Could you check a few things on this model? Use its own coordinates, in mm. Coordinates: 2 decimals unless noted, no trailing zeros. Loops run counter-clockwise (first coordinate to the right, second up) from the corner with the lowest first, then second, coordinate; pieces in that order, holes last. Notation, with made-up numbers: (39.25, 28.5) - (65.25, 28.5) arc R25 cw to (65.25, 66.5) - close; hole circle Ø1 at (70, -34.75). An arc over 180 degrees is marked (long way). One line per question, with ' | ' between items. Start each with the question number.
1. Please list where these lines run through material, in increasing order: L1, parallel to X at y = 8.5, z = 1.3; L2, parallel to X at y = -9, z = 1; L3, parallel to X at y = -1.5, z = 0.1. Write a range as [from, to].
2. I want a section at A-A, the plane x = -5. Write out the boundary of the cut face in (y, z), then the cut area to 3 significant figures.
3. I want a section at B-B, the plane y = 9.78. Write out the boundary of the cut face in (x, z).
4. I want a section at C-C, the plane y = 0. Write out the boundary of the cut face in (x, z).
5. I want a section at D-D, the plane z = 1.3. Count the separate pieces of the cut face and the enclosed holes in it, then the cut area to 3 significant figures.
6. I'm going to push flat-ended pins straight in: P1, Ø3.5, axis at x = 9.78, y = 0, coming from the -Z side; P2, Ø1, axis at y = 9, z = 1, coming from the +X side; P3, Ø0.6, axis at y = -10, z = 1, coming from the +X side. Where does each tip first touch, or does it pass through?
from build123d import *

# Parameters (mm, degrees)
SKETCH1_R           = 17.5
SKETCH1_R_2         = 5.9
SKETCH1_R_3         = 15
BOSS_EXTRUDE1_DEPTH = 2
SKETCH2_R           = 2.25
CUT_EXTRUDE1_DEPTH  = 78.040573726
SKETCH3_R           = 2.4
CUT_EXTRUDE2_DEPTH  = 78.040573726
SKETCH4_W           = 3
SKETCH4_H           = 6
CUT_EXTRUDE3_DEPTH  = 10
SKETCH5_R           = 2.5
CUT_EXTRUDE4_DEPTH  = 78.040573726


with BuildPart() as part:
    # Sketch1 → Boss-Extrude1 (new body)
    # profile 1 of 3: a face of its own
    with BuildSketch(Plane.XY):
        Circle(SKETCH1_R)
        Circle(SKETCH1_R_2, mode=Mode.SUBTRACT)
    # profile 2 of 3: a face of its own
    with BuildSketch(Plane.XY):
        with Locations((-60, 0)):
            Circle(SKETCH1_R_3)
    # profile 3 of 3: a face of its own
    with BuildSketch(Plane.XY):
        with BuildLine():
            Line((-0.729166667, 17.484802429), (-60.625, 14.98697351))
            ThreePointArc((-60.625, 14.98697351), (-49.616720171, 10.825317547), (-45, 0))
            ThreePointArc((-45, 0), (-49.616720171, -10.825317547), (-60.625, -14.98697351))
            Line((-60.625, -14.98697351), (-0.729166667, -17.484802429))
            ThreePointArc((-0.729166667, -17.484802429), (-17.5, 0), (-0.729166667, 17.484802429))
        make_face()
    extrude(amount=BOSS_EXTRUDE1_DEPTH)

    # Sketch2 → Cut-Extrude1 (cut, through all)
    with BuildSketch(Plane.XY.offset(2)):
        with Locations((0, 9.78)):
            Circle(SKETCH2_R)
        with Locations((9.78, 0)):
            Circle(SKETCH2_R)
        with Locations((0, -9.78)):
            Circle(SKETCH2_R)
        with Locations((-9.78, 0)):
            Circle(SKETCH2_R)
    extrude(amount=-CUT_EXTRUDE1_DEPTH, mode=Mode.SUBTRACT)

    # Sketch3 → Cut-Extrude2 (cut, through all)
    with BuildSketch(Plane.XY.offset(2)):
        with Locations((-60, 0)):
            Circle(SKETCH3_R)
    extrude(amount=-CUT_EXTRUDE2_DEPTH, mode=Mode.SUBTRACT)

    # Sketch4 → Cut-Extrude3 (cut)
    with BuildSketch(Plane.XY.offset(2)):
        with Locations((-44.5, -9.405729391)):
            Rectangle(SKETCH4_W, SKETCH4_H)
        with Locations((-44.5, 9.594270609)):
            Rectangle(SKETCH4_W, SKETCH4_H)
    extrude(amount=-CUT_EXTRUDE3_DEPTH, mode=Mode.SUBTRACT)

    # Sketch5 → Cut-Extrude4 (cut, through all)
    with BuildSketch(Plane.XY.offset(2)):
        with Locations((-35.840347269, -8.875222906)):
            Circle(SKETCH5_R)
    extrude(amount=-CUT_EXTRUDE4_DEPTH, mode=Mode.SUBTRACT)


solid = part.part
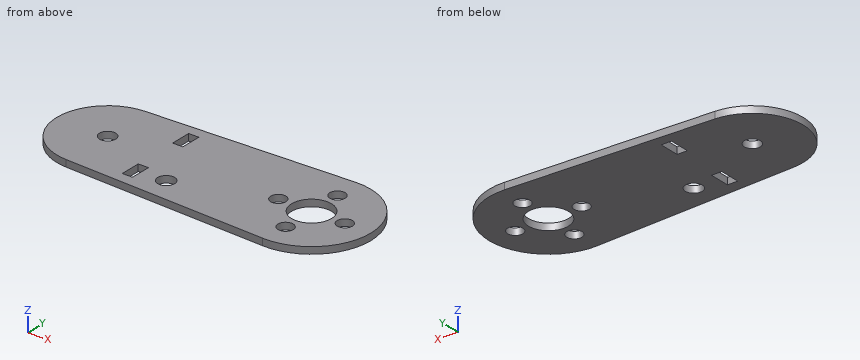
Results are:
1) L1: x = [-72.36, -46], [-43, -1.85], [1.85, 15.3] | L2: x = [-72, -46], [-43, -38.34], [-33.34, -2.11], [2.11, 15.01] | L3: x = [-74.92, -61.87], [-58.13, -11.46], [-8.1, -5.71], [5.71, 8.1], [11.46, 17.44]
2) outline: (-17.31, 0) - (-3.13, 0) - (-3.13, 2) - (-17.31, 2) - close; (3.13, 0) - (17.31, 0) - (17.31, 2) - (3.13, 2) - close | area: 56.7 mm2
3) outline: (-71.37, 0) - (-46, 0) - (-46, 2) - (-71.37, 2) - close; (-43, 0) - (-2.25, 0) - (-2.25, 2) - (-43, 2) - close; (2.25, 0) - (14.51, 0) - (14.51, 2) - (2.25, 2) - close
4) outline: (-75, 0) - (-62.4, 0) - (-62.4, 2) - (-75, 2) - close; (-57.6, 0) - (-12.03, 0) - (-12.03, 2) - (-57.6, 2) - close; (-7.53, 0) - (-5.9, 0) - (-5.9, 2) - (-7.53, 2) - close; (5.9, 0) - (7.53, 0) - (7.53, 2) - (5.9, 2) - close; (12.03, 0) - (17.5, 0) - (17.5, 2) - (12.03, 2) - close
5) separate pieces: 1 | enclosed holes: 9 | area: 2,540 mm2
6) P1: passes through | P2: stops at x = 15.3 | P3: stops at x = 14.57
